Can you work these out from the model? Positions are in its coordinate system, mm. A direction names the side the tool comes from. Give positions to 0.01 mm unless a question says otherwise; leave off trailing zeros. Loops run counter-clockwise (first coordinate to the right, second up) from the corner with the lowest first, then second, coordinate; pieces in that order, holes last. Notation, with made-up numbers: (9, 88.5) -> (54, 88.5) arc R7 cw to (54, 97.5) -> close; hole circle Ø10 at (-20.5, -12.5). An arc over 180 degrees is marked (long way). Use CSV: the item, a comma, the result in double quotes.
from build123d import *

# Parameters (mm, degrees)
BOSS_EXTRUDE1_DEPTH              = 6.35
SKETCH2_W                        = 31.75
SKETCH2_H                        = 9.525
F_2_4_5_TAPPED_HOLE1_D           = 38.1
F_2_4_5_TAPPED_HOLE1_CBORE_D     = 50.8
F_2_4_5_TAPPED_HOLE1_CBORE_DEPTH = 12.7
SKETCH13_R                       = 3.175
CUT_EXTRUDE1_DEPTH               = 66.454301807
CIRPATTERN1_COUNT                = 2
F_6_32_TAPPED_HOLE1_D            = 2.7051
CIRPATTERN2_COUNT                = 6
F_1_4_0_25_DIAMETER_HOLE1_D      = 6.35
F_1_4_0_25_DIAMETER_HOLE2_D      = 6.35


with BuildPart() as part:
    # Sketch1 → Boss-Extrude1 (new body)
    with BuildSketch(Plane(origin=(0, 0, 1.5875), x_dir=(-1, 0, 0), z_dir=(0, 0, -1))):
        with BuildLine():
            Line((38.1, -33.601041651), (38.1, 33.601041651))
            ThreePointArc((38.1, 33.601041651), (0, 50.8), (-38.1, 33.601041651))
            Line((-38.1, 33.601041651), (-38.1, -33.601041651))
            ThreePointArc((-38.1, -33.601041651), (0, -50.8), (38.1, -33.601041651))
        make_face()
    extrude(amount=-BOSS_EXTRUDE1_DEPTH)

    # Sketch2 → Revolve1 (revolve)
    with BuildSketch(Plane(origin=(0, 0, 0), x_dir=(1, 0, 0), z_dir=(0, 1, 0))):
        with Locations((15.875, 3.175)):
            Rectangle(SKETCH2_W, SKETCH2_H)
    revolve(axis=Axis((0, 0, -7.9375), (0, 0, 1)))

    # 2-4.5 Tapped Hole1 (through all)
    with Locations(Plane.XY.offset(7.9375)):
        with Locations((0, 0)):
            CounterBoreHole(F_2_4_5_TAPPED_HOLE1_D / 2, F_2_4_5_TAPPED_HOLE1_CBORE_D / 2, F_2_4_5_TAPPED_HOLE1_CBORE_DEPTH)

    # Sketch13 → Cut-Extrude1 (cut, through all)
    with BuildSketch(Plane.XY.offset(7.9375)):
        with Locations((0, 44.45)):
            Circle(SKETCH13_R)
    cut_extrude1 = extrude(amount=-CUT_EXTRUDE1_DEPTH, mode=Mode.SUBTRACT)

    # CirPattern1: Cut-Extrude1 ×2 about axis
    cirpattern1_axis = Axis((0, 0, 0), (0, 0, 1))
    for i in range(1, CIRPATTERN1_COUNT):
        add(cut_extrude1.rotate(cirpattern1_axis, i * 360 / CIRPATTERN1_COUNT), mode=Mode.SUBTRACT)

    # #6-32 Tapped Hole1 (through all)
    with Locations(Plane.XY.offset(7.9375)):
        with Locations((28.575, 0)):
            f_6_32_tapped_hole1 = Hole(F_6_32_TAPPED_HOLE1_D / 2)

    # CirPattern2: #6-32 Tapped Hole1 ×6 about axis
    cirpattern2_axis = Axis((0, 0, 0), (0, 0, 1))
    for i in range(1, CIRPATTERN2_COUNT):
        add(f_6_32_tapped_hole1.rotate(cirpattern2_axis, i * 360 / CIRPATTERN2_COUNT), mode=Mode.SUBTRACT)

    # 1/4 (0.25) Diameter Hole1 (through all)
    with Locations(Plane.XY.offset(7.9375)):
        with Locations((-19.05, 40.160926284)):
            Hole(F_1_4_0_25_DIAMETER_HOLE1_D / 2)

    # 1/4 (0.25) Diameter Hole2 (through all)
    with Locations(Plane.XY.offset(7.9375)):
        with Locations((19.05, 40.160926284), (19.05, -40.160926284), (-19.05, -40.160926284)):
            Hole(F_1_4_0_25_DIAMETER_HOLE2_D / 2)


solid = part.part
(1) If we section it at D-D, the plane y = -13: Write out the boundary of the cut face in (x, z), then the cut area to 3 significant figures.
Answer sheet:
outline,"(-38.1, 1.59) -> (-28.97, 1.59) -> (-28.97, -7.94) -> (-13.92, -7.94) -> (-13.92, -4.76) -> (-21.82, -4.76) -> (-21.82, 7.94) -> (-38.1, 7.94) -> close; (13.92, -7.94) -> (28.97, -7.94) -> (28.97, 1.59) -> (38.1, 1.59) -> (38.1, 7.94) -> (21.82, 7.94) -> (21.82, -4.76) -> (13.92, -4.76) -> close"
area,"393 mm2"
(2) Will these pins go through, and if not, where does the flat tip stop? pin 1 Ø4.5 at (x, y) = (-14.29, -24.75) entering from -Z; pin 2 Ø8 at (x, z) = (3, -5) entering from +Y; pin 3 Ø5 at (x, y) = (-30, 29.5) entering from -Z; pin 4 Ø1 at (y, z) = (13.5, -6) entering from +X.
Answer sheet:
pin 1,"stops at z = -7.94"
pin 2,"stops at y = 31.75"
pin 3,"stops at z = 1.59"
pin 4,"stops at x = 28.97"
(3) Which directions (+Z, -Z, +X, -X, +Y, -Y) give clear straight access to the entire face, cutting with the end or side of a thin tool? Please do faces 4 (the face through (15.12, -11.59, -6.37)), 5 (the face through (-6.883, -30.995, -3.242)), 6 (the face through (4, 19, -4.762)).
Answer sheet:
face 4,"+Z, -Z"
face 5,"-Z"
face 6,"+Z"
(4) We'd pull the mould along X, two halves only. Please class faces 1 (the face through (1, 35, 1.588)), 2 (the face through (-0.603, 50.796, 4.718)), 3 (the face through (-1.707, -47.127, 4.807)): released by +X, released by -X, zero draft, split by the parting line, or undercut.
Answer sheet:
face 1,"zero draft"
face 2,"split by the parting line"
face 3,"undercut"
(5) If we section it at A-A, the plane x = 0: Give the number of separate pieces and of enclosed holes in the cut face, then the cut area to 3 significant figures.
Answer sheet:
separate pieces,"4"
enclosed holes,"0"
area,"403 mm2"
(6) If we section it at C-C, the plane y = 12: Write out the boundary of the cut face in (x, z).
Answer sheet:
outline,"(-38.1, 1.59) -> (-29.39, 1.59) -> (-29.39, -7.94) -> (-14.8, -7.94) -> (-14.8, -4.76) -> (-22.39, -4.76) -> (-22.39, 7.94) -> (-38.1, 7.94) -> close; (14.8, -7.94) -> (29.39, -7.94) -> (29.39, 1.59) -> (38.1, 1.59) -> (38.1, 7.94) -> (22.39, 7.94) -> (22.39, -4.76) -> (14.8, -4.76) -> close"
(7) If we section it at B-B, the plane y = 0: Write out the boundary of the cut face in (x, z), then the cut area to 3 significant figures.
Answer sheet:
outline,"(-38.1, 1.59) -> (-31.75, 1.59) -> (-31.75, -7.94) -> (-29.93, -7.94) -> (-29.93, 7.94) -> (-38.1, 7.94) -> close; (-27.22, -7.94) -> (-19.05, -7.94) -> (-19.05, -4.76) -> (-25.4, -4.76) -> (-25.4, 7.94) -> (-27.22, 7.94) -> close; (19.05, -7.94) -> (27.22, -7.94) -> (27.22, 7.94) -> (25.4, 7.94) -> (25.4, -4.76) -> (19.05, -4.76) -> close; (29.93, -7.94) -> (31.75, -7.94) -> (31.75, 1.59) -> (38.1, 1.59) -> (38.1, 7.94) -> (29.93, 7.94) -> close"
area,"237 mm2"
(8) If I drill on L1, parallel to Y at x = 0, z = 4 (3 decimals); L2, parallel to X at y = 25, z = -5.75; L3, parallel to X at y = 40, z = 4.5, over which ranges is the centre line in solid material (lowest first)? Write a range as from..to.
Answer sheet:
L1,"y = -50.8..-47.625, -41.275..-25.4, 25.4..41.275, 47.625..50.8"
L2,"x = -19.57..-15.62, -12.96..12.96, 15.62..19.57"
L3,"x = -31.32..-22.22, -15.88..15.88, 22.22..31.32"
